```python
from build123d import *

# Parameters (mm, degrees)
SKETCH_1_R      = 2.1
EXTRUDE_1_DEPTH = 5
SKETCH_2_W      = 57
SKETCH_2_H      = 49.677447992
EXTRUDE_2_DEPTH = 20


with BuildPart() as part:
    # Эскиз1 → Бобышка-Вытянуть1 (new body)
    with BuildSketch(Plane(origin=(0, 0, 0), x_dir=(1, 0, 0), z_dir=(0, 1, 0))):
        with BuildLine():
            Line((-38.25, -41.25), (38.25, -41.25))
            ThreePointArc((38.25, -41.25), (40.371320344, -40.371320344), (41.25, -38.25))
            Line((41.25, -38.25), (41.25, 38.25))
            ThreePointArc((41.25, 38.25), (40.371320344, 40.371320344), (38.25, 41.25))
            Line((38.25, 41.25), (-38.25, 41.25))
            ThreePointArc((-38.25, 41.25), (-40.371320344, 40.371320344), (-41.25, 38.25))
            Line((-41.25, 38.25), (-41.25, -38.25))
            ThreePointArc((-41.25, -38.25), (-40.371320344, -40.371320344), (-38.25, -41.25))
        make_face()
        with Locations((-33, 33)):
            Circle(SKETCH_1_R, mode=Mode.SUBTRACT)
        with Locations((33, 33)):
            Circle(SKETCH_1_R, mode=Mode.SUBTRACT)
        with Locations((33, -33)):
            Circle(SKETCH_1_R, mode=Mode.SUBTRACT)
        with Locations((-33, -33)):
            Circle(SKETCH_1_R, mode=Mode.SUBTRACT)
        with BuildLine():
            Line((-32.1, 2), (-32.1, -2))
            ThreePointArc((-32.1, -2), (-30, -4.1), (-27.9, -2))
            Line((-27.9, -2), (-27.9, 2))
            ThreePointArc((-27.9, 2), (-30, 4.1), (-32.1, 2))
        make_face(mode=Mode.SUBTRACT)
        with BuildLine():
            Line((32.1, -2), (32.1, 2))
            ThreePointArc((32.1, 2), (30, 4.1), (27.9, 2))
            Line((27.9, 2), (27.9, -2))
            ThreePointArc((27.9, -2), (30, -4.1), (32.1, -2))
        make_face(mode=Mode.SUBTRACT)
    extrude(amount=EXTRUDE_1_DEPTH)

    # Эскиз2 → Бобышка-Вытянуть2 (add)
    with BuildSketch(Plane.XZ):
        Rectangle(SKETCH_2_W, SKETCH_2_H)
    extrude(amount=EXTRUDE_2_DEPTH)


solid = part.part
```
Check sheet for the modelled part. Datum: model origin and axes. Units: mm. A direction names the side the tool comes from. Coordinates: 2 decimals unless noted, no trailing zeros. Order: outer loops, then holes, each group sorted by start corner. A loop starts at its lowest first (then second) coordinate and runs counter-clockwise, first axis right, second up. Notation, with made-up numbers: M 23.25,73 L 76.25,73 A27 ccw 76.25,106 Z; hole C 8,84.5 d2. An arc over 180 degrees is marked long. One line per question, with ' | ' between items. Start each with the question number.
Item 1: Sectioned sample at B-B on x = -16. Record the cut outline in (y, z), and give its area (3 significant figures).
Item 2: Gauge pin test, flat ends, axial feed: P1, Ø5, axis at y = -8, z = 4, coming from the -X side; P2, Ø2, axis at x = -23, y = -7, coming from the +Z side; P3, Ø5.5, axis at x = -33, z = 33, coming from the -Y side. Record the tip position at first contact, or that the pin passes through.
Item 3: Sectioned sample at D-D on y = -5.25. Record the cut outline in (x, z), and give its area (3 significant figures).
Item 4: Material ranges on line 1 (Z direction, x = -33, y = 2.95); line 2 (Y direction, x = 31.5, z = 16.5), recorded low to high.
Item 5: Sectioned sample at C-C on z = 33. Record the cut outline in (x, y), and give its area (4 significant figures).
Item 6: Mould release check, pull along X, two halves, no side actions. Record for faces 1 (the flat face through (-28.5, -10, 0)), 2 (the cylindrical face through (-30, 2.5, -4.1)), 3 (the flat face through (1, 2, -41.25)), 4 (the cylindrical face through (31.334, 2.465, -31.722)): pulls with the +X half, pulls with the -X half, needs draft (parallel to the pull), parting line crosses it, or undercut.
Item 7: Access from +Z, -Z, +X, -X, +Y, -Y to the whole of each face (thin tool, end or side, straight path). Record for faces 5 (the flat face through (-32.1, 2, 0)), 6 (the flat face through (0, -10, -24.839)), 7 (the flat face through (0, -10, 24.839)).
Item 8: Sectioned sample at A-A on z = 0. Record the cut outline in (x, y), and give its area (3 significant figures).
Answer below:
1) outline: M -20,-24.84 L 0,-24.84 L 0,-41.25 L 5,-41.25 L 5,41.25 L 0,41.25 L 0,24.84 L -20,24.84 Z | area: 1,410 mm^2
2) P1: stops at x = -28.5 | P2: stops at z = 24.84 | P3: stops at y = 0
3) outline: M -28.5,-24.84 L 28.5,-24.84 L 28.5,24.84 L -28.5,24.84 Z | area: 2,830 mm^2
4) line 1: z = -41.25 to -35.1, -30.9 to 30.9, 35.1 to 41.25 | line 2: y = 0 to 5
5) outline: M -41.25,0 L -35.1,0 L -35.1,5 L -41.25,5 Z; M -30.9,0 L 30.9,0 L 30.9,5 L -30.9,5 Z; M 35.1,0 L 41.25,0 L 41.25,5 L 35.1,5 Z | area: 370.5 mm^2
6) face 1: pulls with the -X half | face 2: undercut | face 3: needs draft | face 4: undercut
7) face 5: +Y, -Y | face 6: -Z, +X, -X, -Y | face 7: +Z, +X, -X, -Y
8) outline: M -41.25,0 L -32.1,0 L -32.1,5 L -41.25,5 Z; M -28.5,-20 L 28.5,-20 L 28.5,0 L 27.9,0 L 27.9,5 L -27.9,5 L -27.9,0 L -28.5,0 Z; M 32.1,0 L 41.25,0 L 41.25,5 L 32.1,5 Z | area: 1,510 mm^2
